Build history of the part. All positions in model axes, mm. Face numbers are marked on the shaded views. Round coordinates to 2 decimals unless told otherwise and drop trailing zeros. Write each loop counter-clockwise with the first axis right and the second up, starting at its lowest first coordinate (ties: lowest second). Pieces come first, ordered by that corner, then holes. Notation, with made-up numbers: M 58,74.25 L 102,74.25 A20 ccw 102,85.25 Z; hole C 9,26 d7. An arc over 180 degrees is marked long. Write item = value, one per line.
from build123d import *

# Parameters (mm, degrees)
BOSS_EXTRUDE1_DEPTH = 13
SKETCH2_W           = 10
SKETCH2_H           = 8
CUT_EXTRUDE1_DEPTH  = 23
FILLET2_R           = 0.8
FILLET3_R           = 0.4


with BuildPart() as part:
    # Sketch1 → Boss-Extrude1 (new body)
    # profile 1 of 9: a face of its own
    with BuildSketch(Plane(origin=(0, 0, 0), x_dir=(1, 0, 0), z_dir=(0, 1, 0))):
        with BuildLine():
            Line((0, 51.69999999999999), (0, 52.99999999999999))
            ThreePointArc((-9.3e-16, 52.999999999999986), (-4.000000000000001, 48.999999999999986), (0, 44.999999999999986))
            ThreePointArc((0, 44.99999999999999), (40.783850416649216, 19.017821778331506), (34.47199994035405, -28.925442435894198))
            Line((34.47199994035406, -28.9254424358942), (35.888260603401996, -30.337605930077153))
            Line((35.888260603401996, -30.337605930077153), (36.00408882659202, -30.211017655267263))
            ThreePointArc((36.00408882659201, -30.211017655267256), (46.250188794991274, -3.909012128546492), (40.31112943915424, 23.686379393552375))
            ThreePointArc((40.31112943915424, 23.686379393552375), (24.563687739130117, 40.824426362915915), (2.690955139008132, 48.77918233801223))
            ThreePointArc((2.6909551390081288, 48.77918233801222), (-1.985725017136943, 47.17054758019878), (2.055e-14, 51.69999999999999))
        make_face()
    # profile 2 of 9: a face of its own
    with BuildSketch(Plane(origin=(0, 0, 0), x_dir=(1, 0, 0), z_dir=(0, 1, 0))):
        with BuildLine():
            Line((50.82068164403521, 29.47855622552852), (0, 52.99999999999999))
            Line((0, 52.99999999999999), (0, 51.69999999999999))
            ThreePointArc((2.115e-14, 51.69999999999999), (1.909188309203686, 50.90918830920366), (2.7, 48.999999999999986))
            ThreePointArc((2.7, 48.999999999999986), (2.6977378370888774, 48.88949858671026), (2.6909551390081288, 48.77918233801222))
            ThreePointArc((2.690955139008132, 48.77918233801223), (24.563687739130117, 40.824426362915915), (40.31112943915424, 23.686379393552375))
            Line((40.311129439154236, 23.68637939355237), (50.82068164403521, 29.47855622552852))
        make_face()
    # profile 3 of 9: a face of its own
    with BuildSketch(Plane(origin=(0, 0, 0), x_dir=(1, 0, 0), z_dir=(0, 1, 0))):
        Polygon((21.766625661572498, -44.50021256055632), (35.888260603401996, -30.337605930077153), (34.47199994035406, -28.9254424358942), (20.350364998524487, -43.08804906637342), align=None)
    # profile 4 of 9: a face of its own
    with BuildSketch(Plane(origin=(0, 0, 0), x_dir=(1, 0, 0), z_dir=(0, 1, 0))):
        Polygon((34.83733232049475, -37.056649741824835), (33.063933615036056, -33.170127256173025), (30.23960662667018, -36.00264858226883), (34.13125057340328, -37.76478007334881), (35.5475112364512, -39.17694356753177), (37.32090994190985, -43.063466053183646), (40.145236930275736, -40.230944727087746), (36.25359298354269, -38.468813236007804), align=None)
    # profile 5 of 9: a face of its own
    with BuildSketch(Plane(origin=(0, 0, 0), x_dir=(1, 0, 0), z_dir=(0, 1, 0))):
        Polygon((51.446642052604496, -31.729283579935103), (30.26418963986006, -52.973193525654075), (28.84792897681213, -51.56103003147111), (50.03038138955656, -30.317120085752126), align=None)
    # profile 6 of 9: a face of its own
    with BuildSketch(Plane(origin=(0, 0, 0), x_dir=(1, 0, 0), z_dir=(0, 1, 0))):
        Polygon((23.17878915575541, -43.08395189750844), (22.47270740866399, -43.792082229032346), (29.270758591293983, -50.57046700111064), (34.50173196536596, -43.07678265401291), (35.9087464477269, -44.47972671623149), (36.61482819481838, -43.77159638470753), (29.81677701218832, -36.993211612629345), (24.585803638116356, -44.48689595972706), align=None)
        Polygon((32.77765265760353, -41.35769101853769), (28.12789854731734, -48.01874377151343), (27.490581248945773, -47.38327019913109), (32.14033535923197, -40.722217446155355), align=None, mode=Mode.SUBTRACT)
        Polygon((31.596954354536543, -40.1804084146089), (26.947200244250347, -46.84146116758463), (26.309882945878776, -46.20598759520231), (30.959637056164965, -39.54493484222657), align=None, mode=Mode.SUBTRACT)
        Polygon((33.95835096067053, -42.534973622466474), (29.308596850384333, -49.196026375442216), (28.671279552012766, -48.560552803059885), (33.321033662298966, -41.89950005008415), align=None, mode=Mode.SUBTRACT)
        Polygon((30.416256051469542, -39.00312581068011), (25.766501941183353, -45.664178563655845), (25.129184642811783, -45.02870499127351), (29.778938753097975, -38.36765223829777), align=None, mode=Mode.SUBTRACT)
    # profile 7 of 9: a face of its own
    with BuildSketch(Plane(origin=(0, 0, 0), x_dir=(1, 0, 0), z_dir=(0, 1, 0))):
        Polygon((27.435765482629172, -52.977290694519034), (28.84792897681213, -51.56103003147111), (30.26418963986006, -52.973193525654075), (27.439862651494142, -55.805714851749926), (23.899210993874338, -52.27530611629255), (21.074884005508324, -55.10782744238849), (19.658623342460395, -53.69566394820553), (23.895113825009364, -49.446881959061656), align=None)
    # profile 8 of 9: a face of its own
    with BuildSketch(Plane(origin=(0, 0, 0), x_dir=(1, 0, 0), z_dir=(0, 1, 0))):
        Polygon((19.658623342460395, -53.69566394820553), (21.07078683664336, -52.27940328515759), (19.654526173595425, -50.86723979097463), align=None)
    # profile 9 of 9: a face of its own
    with BuildSketch(Plane(origin=(0, 0, 0), x_dir=(1, 0, 0), z_dir=(0, 1, 0))):
        Polygon((20.350364998524487, -43.08804906637342), (14.701711021792637, -48.753091718565145), (16.11797168484057, -50.165255212748114), (21.766625661572498, -44.50021256055632), align=None)
    extrude(amount=BOSS_EXTRUDE1_DEPTH)

    # Sketch2 → Cut-Extrude1 (cut)
    with BuildSketch(Plane(origin=(-10.69214872852209, 0, 10.723170305733387), x_dir=(0.7081303315239577, 0, 0.7060817470914894), z_dir=(-0.7060817470914894, 0, 0.7081303315239577))):
        with Locations((51.834395676587455, 6.499999999999998)):
            Rectangle(SKETCH2_W, SKETCH2_H)
    extrude(amount=-CUT_EXTRUDE1_DEPTH, mode=Mode.SUBTRACT)

    # Fillet2
    fillet2_edges = [part.edges().sort_by_distance(p)[0] for p in [
        (35.5475112364512, 11.75, 39.17694356753177),
        (34.13125057340328, 11.75, 37.76478007334881),
        (30.23960662667018, 11.75, 36.00264858226883),
        (37.32090994190983, 11.75, 43.06346605318363),
        (50.03038138955656, 6.5, 30.317120085752126),
        (51.446642052604496, 6.5, 31.729283579935103),
        (27.439862651494142, 6.5, 55.805714851749926),
        (21.074884005508324, 6.5, 55.10782744238849),
        (19.658623342460395, 6.5, 53.69566394820553),
        (23.895113825009364, 6.5, 49.446881959061656),
        (27.435765482629172, 6.5, 52.977290694519034),
        (16.11797168484057, 6.5, 50.165255212748114),
        (14.701711021792637, 6.5, 48.753091718565145),
        (50.82068164403521, 6.5, -29.47855622552852),
        (40.31112943915424, 6.5, -23.68637939355238),
        (33.063933615036056, 11.75, 33.170127256173025),
        (34.83733232049475, 11.75, 37.056649741824835),
        (36.25359298354269, 11.75, 38.468813236007804),
        (40.14523693027576, 11.75, 40.23094472708776),
        (33.063933615036056, 1.2499999999999993, 33.170127256173025),
        (34.83733232049475, 1.2499999999999993, 37.056649741824835),
        (36.25359298354269, 1.2499999999999993, 38.468813236007804),
        (40.14523693027576, 1.2499999999999993, 40.23094472708776),
        (30.23960662667018, 1.2499999999999993, 36.00264858226883),
        (37.32090994190983, 1.2499999999999993, 43.06346605318363),
    ]]
    fillet(fillet2_edges, radius=FILLET2_R)

    # Fillet3
    fillet3_edges = [part.edges().sort_by_distance(p)[0] for p in [
        (23.17878915575541, 11.75, 43.08395189750844),
        (29.81677701218832, 11.75, 36.993211612629345),
        (36.61482819481838, 11.75, 43.77159638470753),
        (35.9087464477269, 11.75, 44.47972671623149),
        (29.270758591293983, 11.75, 50.57046700111064),
        (22.472707408664043, 11.75, 43.7920822290324),
        (35.9087464477269, 1.2499999999999993, 44.47972671623149),
        (29.270758591293983, 1.2499999999999993, 50.57046700111064),
        (22.472707408664043, 1.2499999999999993, 43.7920822290324),
        (23.17878915575541, 1.2499999999999993, 43.08395189750844),
        (29.81677701218832, 1.2499999999999993, 36.993211612629345),
        (36.61482819481838, 1.2499999999999993, 43.77159638470753),
    ]]
    fillet(fillet3_edges, radius=FILLET3_R)


solid = part.part
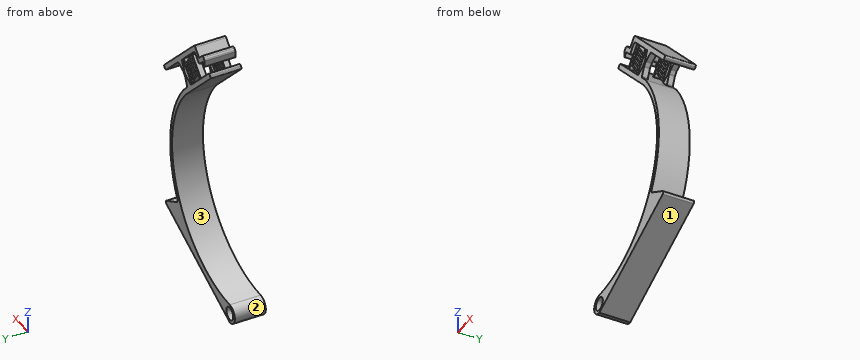
1. Band-saw the part on D-D (z = 4). List the corners of the cut face in (x, y).
Responses:
outline = M 44.82,0 L 46.24,0 L 46.24,13 L 44.82,13 Z
2. Band-saw the part on C-C (x = 10). List the corners of the cut face in (y, z), plus the area to 3 significant figures.
Responses:
outline = M 0,-48.37 L 13,-48.37 L 13,-43.87 L 0,-43.87 Z
area = 58.5 mm²
3. Mould opens along Z. For the marked faces 1, 2 and 3 say: pulls with the +Z half, pulls with the -Z half, needs draft (parallel to the pull), parting line crosses it, or undercut.
Responses:
face_1 = pulls with the -Z half
face_2 = parting line crosses it
face_3 = undercut
4. Band-saw the part on A-A (y = 8.75). Count the separate pieces of the cut face and the enclosed holes in it, plus the area to 3 significant figures.
Responses:
separate_pieces = 2
enclosed_holes = 1
area = 520 mm²
5. Band-saw the part on B-B (z = -49). List the corners of the cut face in (x, y), plus the area to 3 significant figures.
Responses:
outline = M -4,0 L -2.7,0 L -2.7,13 L -4,13 Z; M 2.7,0 L 8.64,0 L 8.64,13 L 2.7,13 Z
area = 94.2 mm²
6. Flat gauge pins, fed straight in: pin 1 (1.5 mm diameter, centred on x = 38, y = 10.5, fed in from +Z); pin 2 (5 mm diameter, centred on x = 0, z = -49, fed in from -Y); pin 3 (3 mm diameter, centred on y = 10, z = -39.5, fed in from +X). Where does each tip first touch, or does it go through?
Responses:
pin_1 = 45.97
pin_2 = through
pin_3 = 32.41
7. Probe probe 1 along Z at (x, y) = (34.5, 10.75); probe 2 along Z at (x, y) = (23.5, 4.75); probe 3 along Z at (x, y) = (39.5, 11.5). List the from-to ranges inside material, lowest first.
Responses:
probe_1 = -37.03 to -28.89, 28.89 to 31.73, 36.32 to 38.13, 41.66 to 43.08, 45.89 to 48.73
probe_2 = -42.12 to -38.38, 39.93 to 42.76, 49.88 to 52.68
probe_3 = -34.72 to -21.56, 21.56 to 25.1, 39.94 to 43.71
